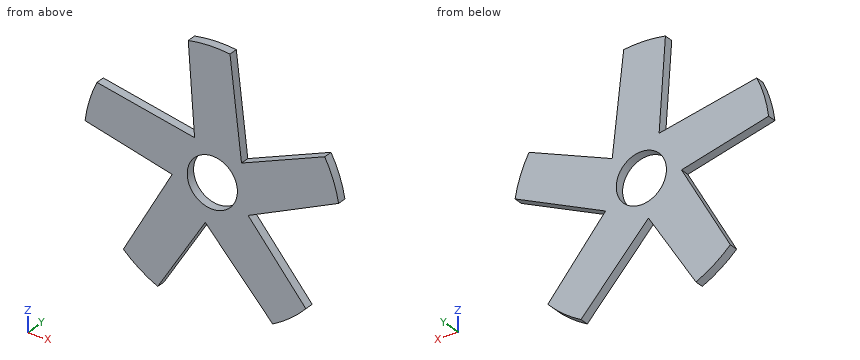
from build123d import *

# Parameters (mm, degrees)
F0_R            = 115
F0_R_2          = 22.5
F1_DEPTH        = 8
F3_DEPTH        = 25
F3_COPIES_COUNT = 5


# Not quite as in the source:
# - a pattern or mirror of a feature is missing from the dataset's text; its kind, count and spacing are read off the source's solid


with BuildPart() as f1:
    # F0 (on Front) → F1 (new body)
    with BuildSketch(Plane.XZ):
        Circle(F0_R)
        Circle(F0_R_2, mode=Mode.SUBTRACT)
    extrude(amount=F1_DEPTH)

    # F2 (on face) → F3 (cut)
    with BuildSketch(Plane.XZ.offset(8)):
        Polygon((100.7627065135, 144.0385852402), (15.8349641698, 113.9045824791), (26.1514205486, 25.2313297242), (100.7627065135, 55.4245160203), align=None)
    f3 = extrude(amount=-F3_DEPTH, mode=Mode.SUBTRACT)

    # F3_copies: F3 ×5 about axis
    f3_copies_axis = Axis((0, 0, 0), (0, 1, 0))
    for i in range(1, F3_COPIES_COUNT):
        add(f3.rotate(f3_copies_axis, i * 360 / F3_COPIES_COUNT), mode=Mode.SUBTRACT)


solid = f1.part
Here's how the part is built. I have some questions about the finished solid (model axes, mm). Round coordinates to 2 decimals unless told otherwise and drop trailing zeros. Loops run counter-clockwise (first coordinate to the right, second up) from the corner with the lowest first, then second, coordinate; pieces in that order, holes last. Notation, with made-up numbers: (85.25, -3.5) - (132.25, -3.5) arc R5 ccw to (132.25, 3.5) - close; hole circle Ø8 at (54.5, 62). An arc over 180 degrees is marked (long way). One line per question, with ' | ' between items. Start each with the question number.
Q1. Will these pins go through, and if not, where does the flat tip stop? pin 1 (2 mm diameter, centred on x = 29, y = -4, fed in from -Z); pin 2 (1 mm diameter, centred on x = -41.5, y = -4, fed in from -Z); pin 3 (1 mm diameter, centred on x = -38.5, y = -3, fed in from -Z).
Q2. Please list where these lines run through material, in increasing order: line 1 (Z direction, x = 0, y = -3); line 2 (Z direction, x = -51.5, y = -2.25); line 3 (X direction, y = -1.75, z = -17). Write a range as [from, to].
Q3. I want a section at B-B (x = 38.5). Write out the boundary of the cut face in (y, z).
Q4. I want a section at D-D (x = -29.5). Write out the boundary of the cut face in (y, z), then the cut area to 3 significant figures.
Q5. I want a section at C-C (z = 0). Write out the boundary of the cut face in (x, y), then the cut area to 3 significant figures.
Q6. I want a section at A-A (y = -4.25). Write out the boundary of the cut face in (x, z), then the cut area to 3 significant figures.
Response values:
1) pin 1: stops at z = -75.24 | pin 2: stops at z = -92.94 | pin 3: stops at z = -88.14
2) line 1: z = [-42.66, -22.5], [22.5, 115] | line 2: z = [-102.82, -32.61], [-1.18, 39.82] | line 3: x = [-42.72, -14.74], [14.74, 32.24]
3) outline: (-8, -84.47) - (0, -84.47) - (0, -24.72) - (-8, -24.72) - close; (-8, -14.13) - (0, -14.13) - (0, 30.23) - (-8, 30.23) - close
4) outline: (-8, -72.92) - (0, -72.92) - (0, 35.4) - (-8, 35.4) - close | area: 867 mm²
5) outline: (-56.25, -8) - (-22.5, -8) - (-22.5, 0) - (-56.25, 0) - close; (22.5, -8) - (69.31, -8) - (69.31, 0) - (22.5, 0) - close | area: 645 mm²
6) outline: (-114.1, 14.39) - (-35.99, -5.04) - (-79.76, -82.84) arc R115 ccw to (-48.94, -104.07) - (-6.33, -35.78) - (54.14, -101.46) arc R115 ccw to (83.85, -78.7) - (32.08, -17.07) - (113.22, 20.14) arc R115 ccw to (100.76, 55.42) - (26.15, 25.23) - (15.83, 113.9) arc R115 ccw to (-21.57, 112.96) - (-15.92, 32.67) - (-103.44, 50.26) arc R115 ccw to start; hole circle Ø45 at (0, 0) | area: 18,400 mm²
